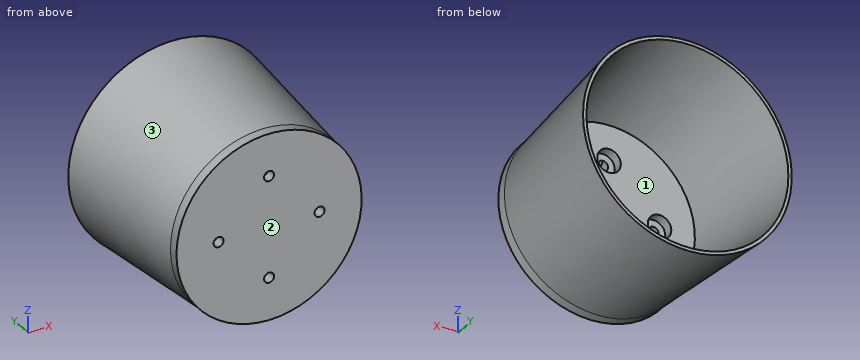
from build123d import *
from build123d.topology import SkipClean

# Parameters (mm, degrees)
SKETCH1_R           = 27.5
SKETCH3_R           = 31
SKETCH3_4_R         = 30
SKETCH1_4_R         = 26.5
SKETCH4_R           = 27.5
SKETCH4_R_2         = 1.5
BOSS_EXTRUDE1_DEPTH = 3
BOSS_EXTRUDE2_START = 6
SKETCH6_R           = 25.5
SKETCH6_R_2         = 1.5
BOSS_EXTRUDE2_DEPTH = 6
SKETCH7_R           = 3.5
CUT_EXTRUDE1_DEPTH  = 3


with BuildPart() as part:
    # Sketch1 → Loft1 section 0
    with BuildSketch(Plane(origin=(0, 0, 0), x_dir=(1, 0, 0), z_dir=(0, 1, 0))):
        Circle(SKETCH1_R)
    # Sketch3 → Loft1 section 1
    with BuildSketch(Plane(origin=(0, 45, 0), x_dir=(1, 0, 0), z_dir=(0, 1, 0))):
        Circle(SKETCH3_R)
    loft()

    # Sketch3<4> → Cut-Loft1 section 0
    with BuildSketch(Plane(origin=(0, 45, 0), x_dir=(1, 0, 0), z_dir=(0, 1, 0))):
        Circle(SKETCH3_4_R)
    # Sketch1<4> → Cut-Loft1 section 1
    with BuildSketch(Plane(origin=(0, 0, 0), x_dir=(1, 0, 0), z_dir=(0, 1, 0))):
        Circle(SKETCH1_4_R)
    loft(mode=Mode.SUBTRACT)

    # Sketch4 → Boss-Extrude1 (add)
    with BuildSketch(Plane.XZ):
        with Locations(Location((0, 0, 0), (0, 0, 270))):
            Circle(SKETCH4_R)
        with Locations(Location((0, 15, 0), (0, 0, 270))):
            Circle(SKETCH4_R_2, mode=Mode.SUBTRACT)
        with Locations(Location((15, 0, 0), (0, 0, 270))):
            Circle(SKETCH4_R_2, mode=Mode.SUBTRACT)
        with Locations(Location((0, -15, 0), (0, 0, 270))):
            Circle(SKETCH4_R_2, mode=Mode.SUBTRACT)
        with Locations(Location((-15, 0, 0), (0, 0, 270))):
            Circle(SKETCH4_R_2, mode=Mode.SUBTRACT)
    extrude(amount=BOSS_EXTRUDE1_DEPTH)

    # Sketch6 → Boss-Extrude2 (add)
    with SkipClean():  # the faces are left unmerged after this step: merging them gives an invalid solid
        with BuildSketch(Plane(origin=(0, 0, 0), x_dir=(1, 0, 0), z_dir=(0, 1, 0)).offset(BOSS_EXTRUDE2_START)):
            with Locations(Location((0, 0, 0), (0, 0, 90))):
                Circle(SKETCH6_R)
            with Locations(Location((0, 15, 0), (0, 0, 270))):
                Circle(SKETCH6_R_2, mode=Mode.SUBTRACT)
            with Locations(Location((15, 0, 0), (0, 0, 270))):
                Circle(SKETCH6_R_2, mode=Mode.SUBTRACT)
            with Locations(Location((0, -15, 0), (0, 0, 270))):
                Circle(SKETCH6_R_2, mode=Mode.SUBTRACT)
            with Locations(Location((-15, 0, 0), (0, 0, 270))):
                Circle(SKETCH6_R_2, mode=Mode.SUBTRACT)
        extrude(amount=-BOSS_EXTRUDE2_DEPTH)

    # Sketch7 → Cut-Extrude1 (cut)
    with SkipClean():  # the faces are left unmerged after this step: merging them gives an invalid solid
        with BuildSketch(Plane(origin=(0, 6, 0), x_dir=(1, 0, 0), z_dir=(0, 1, 0))):
            with Locations(Location((0, 15, 0), (0, 0, 270))):
                Circle(SKETCH7_R)
            with Locations(Location((15, 0, 0), (0, 0, 270))):
                Circle(SKETCH7_R)
            with Locations(Location((0, -15, 0), (0, 0, 270))):
                Circle(SKETCH7_R)
            with Locations(Location((-15, 0, 0), (0, 0, 270))):
                Circle(SKETCH7_R)
        extrude(amount=-CUT_EXTRUDE1_DEPTH, mode=Mode.SUBTRACT)


solid = part.part
Read the model definition and answer for the solid it produces. Units are mm, in the model's axes. Face numbers are marked on the shaded views. Round coordinates to 2 decimals unless told otherwise and drop trailing zeros. Order: outer loops, then holes, each group sorted by start corner. A loop starts at its lowest first (then second) coordinate and runs counter-clockwise, first axis right, second up. Notation, with made-up numbers: (86.5, 88) - (135.5, 88) arc R8 ccw to (135.5, 100) - close; hole circle Ø9 at (-12, 22.5). An arc over 180 degrees is marked (long way). Use one line per item in the form item = value. Start each with the question number.
(1) Determine the mould class of the marked faces 1, 2 and 3 for opening direction X: +X half, -X half, draft (parallel to the pull), parting line (faces both ways), or undercut.
(2) Flat-ended cylindrical pins translate along their axes: pin 1 Ø7.5 at (x, z) = (1, -16) entering from +Y; pin 2 Ø1.5 at (x, y) = (8.5, 27) entering from -Z; pin 3 Ø5.5 at (x, z) = (0, -15) entering from +Y. Find the tip coordinate at first contact, or state that the pin passes through.
(3) The part is cut by section D-D (y = 15). Give the vertices of the cut face in (x, z).
(4) Find the intervals of material crossed by line 1 along Z through (x, y) = (0, -2); line 2 along X through (y, z) = (2, 0); line 3 along X through (y, z) = (4, 0), in increasing order. Write a range as from..to.
(5) The part is cut by section C-C (y = 9). Give the vertices of the cut face in (x, z).
Checked values:
q1.face_1 = undercut
q1.face_2 = draft
q1.face_3 = parting line
q2.pin_1 = 6
q2.pin_2 = -28.58
q2.pin_3 = 3
q3.outline = circle Ø57.33 at (0, 0); hole circle Ø55.33 at (0, 0)
q4.line_1 = -27.5..-16.5, -13.5..13.5, 16.5..27.5
q4.line_2 = -27.66..-26.66, -25.5..-16.5, -13.5..13.5, 16.5..25.5, 26.66..27.66
q4.line_3 = -27.81..-26.81, -25.5..-18.5, -11.5..11.5, 18.5..25.5, 26.81..27.81
q5.outline = circle Ø56.4 at (0, 0); hole circle Ø54.4 at (0, 0)
